from build123d import *

# Parameters (mm, degrees)
F0_W     = 127
F0_H     = 76.2
F1_DEPTH = 50.8
F2_R     = 25.4
F3_DEPTH = 25.4
F4_R     = 12.7
F5_SIZE  = 3.175


with BuildPart() as f1:
    # F0 (on Top) → F1 (new body)
    with BuildSketch(Plane.XY):
        Rectangle(F0_W, F0_H)
    extrude(amount=F1_DEPTH)

    # F2 (on face) → F3 (cut)
    with BuildSketch(Plane.XY.offset(50.8)):
        Circle(F2_R)
    extrude(amount=-F3_DEPTH, mode=Mode.SUBTRACT)

    # F4
    f4_edges = [f1.edges().sort_by_distance(p)[0] for p in [
        (-63.5, -38.1, 25.4),
        (63.5, -38.1, 25.4),
        (63.5, 38.1, 25.4),
        (-63.5, 38.1, 25.4),
    ]]
    fillet(f4_edges, radius=F4_R)

    # F5
    f5_edges = [f1.edges().sort_by_distance(p)[0] for p in [
        (63.5, 0, 50.8),
        (59.780256, -34.380256, 50.8),
        (59.780256, 34.380256, 50.8),
        (0, -38.1, 50.8),
        (0, 38.1, 50.8),
        (-59.780256, -34.380256, 50.8),
        (-59.780256, 34.380256, 50.8),
        (-63.5, 0, 50.8),
        (-25.4, 0, 50.8),
    ]]
    chamfer(f5_edges, length=F5_SIZE)


solid = f1.part
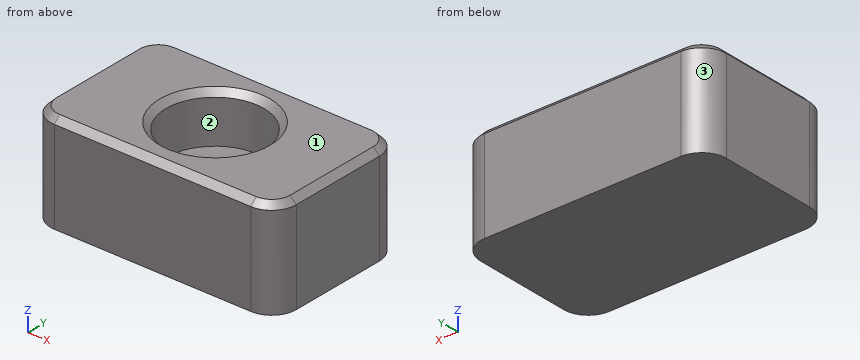
Could you check a few things on this model? Use its own coordinates, in mm. Face numbers are marked on the shaded views. Round coordinates to 2 decimals unless told otherwise and drop trailing zeros. Write each loop counter-clockwise with the first axis right and the second up, starting at its lowest first coordinate (ties: lowest second). Pieces come first, ordered by that corner, then holes. Notation, with made-up numbers: (-12, 76.25) -> (18, 76.25) arc R24 ccw to (18, 86.25) -> close; hole circle Ø1 at (36, 74.25). An arc over 180 degrees is marked (long way). Use a Markdown table: item, result.
1. Please list where these lines run through material, in increasing order: probe 1 along Y at (x, z) = (0, 36); probe 2 along X at (y, z) = (-22, 34); probe 3 along X at (y, z) = (-4, 27).
Answer key:
| item | result |
|---|---|
| probe 1 | y = -38.1 to -25.4, 25.4 to 38.1 |
| probe 2 | x = -63.5 to -12.69, 12.69 to 63.5 |
| probe 3 | x = -63.5 to -25.08, 25.08 to 63.5 |
2. If we section it at B-B (y = 0): List the corners of the cut face in (x, z) for me (3 decimals).
Answer key:
| item | result |
|---|---|
| outline | (-63.5, 0) -> (63.5, 0) -> (63.5, 47.625) -> (60.325, 50.8) -> (28.575, 50.8) -> (25.4, 47.625) -> (25.4, 25.4) -> (-25.4, 25.4) -> (-25.4, 47.625) -> (-28.575, 50.8) -> (-60.325, 50.8) -> (-63.5, 47.625) -> close |
3. If we section it at C-C (x = 0): List the corners of the cut face in (y, z) for me (3 decimals), then the cut area to 3 significant figures.
Answer key:
| item | result |
|---|---|
| outline | (-38.1, 0) -> (38.1, 0) -> (38.1, 47.625) -> (34.925, 50.8) -> (28.575, 50.8) -> (25.4, 47.625) -> (25.4, 25.4) -> (-25.4, 25.4) -> (-25.4, 47.625) -> (-28.575, 50.8) -> (-34.925, 50.8) -> (-38.1, 47.625) -> close |
| area | 2,560 mm^2 |
4. If we section it at A-A (z = 41): List the corners of the cut face in (x, y) for me, then the cut area to 3 significant figures.
Answer key:
| item | result |
|---|---|
| outline | (-63.5, -25.4) arc R12.7 ccw to (-50.8, -38.1) -> (50.8, -38.1) arc R12.7 ccw to (63.5, -25.4) -> (63.5, 25.4) arc R12.7 ccw to (50.8, 38.1) -> (-50.8, 38.1) arc R12.7 ccw to (-63.5, 25.4) -> close; hole circle Ø50.8 at (0, 0) |
| area | 7,510 mm^2 |
5. For pin 1 Ø1 at (y, z) = (30, 24.5) entering from +X; pin 2 Ø4 at (x, y) = (24, 5) entering from +Z; pin 3 Ø15 at (x, y) = (10.5, 9) entering from +Z, each with a flat end and sliding along its axis, tell me the tip position at first contact or that it passes through.
Answer key:
| item | result |
|---|---|
| pin 1 | stops at x = 62.82 |
| pin 2 | stops at z = 48.74 |
| pin 3 | stops at z = 25.4 |
6. We'd pull the mould along X, two halves only. Please class the marked faces 1, 2 and 3: +X half, -X half, draft (parallel to the pull), parting line (faces both ways), or undercut.
Answer key:
| item | result |
|---|---|
| face 1 | draft |
| face 2 | undercut |
| face 3 | -X half |
